```python
from build123d import *

# Parameters (mm, degrees)
SKETCH_1_R          = 27
EXTRUDE_1_DEPTH     = 45
SKETCH_2_R          = 11
CUT_EXTRUDE_1_DEPTH = 20
CUT_EXTRUDE_2_DEPTH = 20


with BuildPart() as part:
    # 草图1 → 凸台-拉伸1 (new body)
    with BuildSketch(Plane(origin=(0, 0, 0), x_dir=(1, 0, 0), z_dir=(0, 1, 0))):
        with Locations(Location((0, 0, 0), (0, 0, 90))):
            Circle(SKETCH_1_R)
    extrude(amount=EXTRUDE_1_DEPTH)

    # 草图2 → 切除-拉伸1 (cut)
    with BuildSketch(Plane(origin=(0, 45, 0), x_dir=(1, 0, 0), z_dir=(0, 1, 0))):
        with Locations(Location((0, 0, 0), (0, 0, 270))):
            Circle(SKETCH_2_R)
    extrude(amount=-CUT_EXTRUDE_1_DEPTH, mode=Mode.SUBTRACT)

    # 草图3 → 切除-拉伸2 (cut)
    with BuildSketch(Plane.XZ):
        with BuildLine():
            Line((-2.6, 10.2), (2.6, 10.2))
            Line((2.6, 10.2), (2.6, 6.499230724))
            ThreePointArc((2.6, 6.499230724), (0, -7), (-2.6, 6.499230724))
            Line((-2.6, 6.499230724), (-2.6, 10.2))
        make_face()
    extrude(amount=-CUT_EXTRUDE_2_DEPTH, mode=Mode.SUBTRACT)


solid = part.part
```
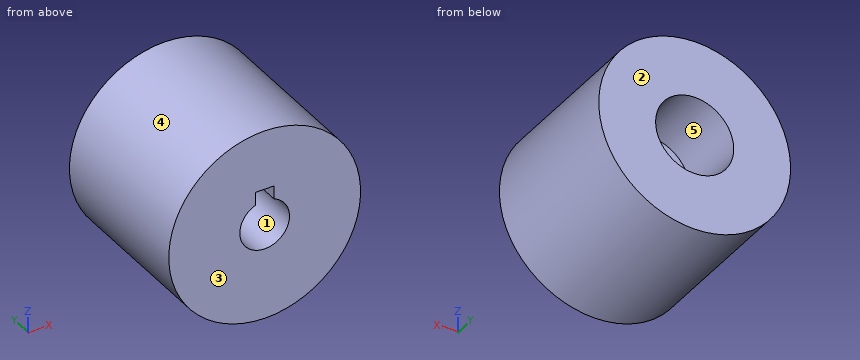
Work out the finished part from the listing and answer in its coordinate system (mm). Face numbers are marked on the shaded views. A direction names the side the tool comes from. Give positions to 0.01 mm unless a question says otherwise; leave off trailing zeros. Loops run counter-clockwise (first coordinate to the right, second up) from the corner with the lowest first, then second, coordinate; pieces in that order, holes last. Notation, with made-up numbers: (75.5, -18) - (123.5, -18) arc R26 cw to (123.5, 9) - close; hole circle Ø3 at (35, 39). An arc over 180 degrees is marked (long way). Use CSV: the item, a comma, the result in double quotes. Start each with the question number.
(1) Determine the mould class of the marked faces 3, 4 and 5 for opening direction X: released by +X, released by -X, zero draft, split by the parting line, or undercut.
(2) Find section C-C, the plane y = 14. Determine the outline of the cut face in (x, z).
(3) Find section D-D, the plane y = 36.5. Determine the outline of the cut face in (x, z).
(4) Find section A-A, the plane z = 0. Determine the outline of the cut face in (x, y), plus the area to 3 significant figures.
(5) Find the intervals of material crossed by L1, parallel to X at y = 37.5, z = 0; L2, parallel to X at y = 11.25, z = 0; L3, parallel to Y at x = -7, z = -4, in increasing order.
(6) Each of these flat-tipped pins is pushed along its axis until it touches: pin 1 (1.9 mm diameter, centred on y = 11.5, z = 8, fed in from -X); pin 2 (4 mm diameter, centred on x = -4, y = 22, fed in from -Z); pin 3 (3 mm diameter, centred on y = 6.5, z = -2.5, fed in from -X). Where does it stop, or does it pass through?
(7) A tool of negligible diameter and unlimited length cuts with its end or side. For the marked faces 1 and 2, from which of +Z, -Z, +X, -X, +Y, -Y can it reach the whole face along a straight path? Write none if from no direction.
(8) Find section B-B, the plane x = 0. Determine the outline of the cut face in (y, z), plus the area to 3 significant figures.
Results found:
1,face 3,"zero draft"
1,face 4,"split by the parting line"
1,face 5,"undercut"
2,outline,"circle Ø54 at (0, 0); hole (-2.6, 6.5) arc R7 ccw (long way) to (2.6, 6.5) - (2.6, 10.2) - (-2.6, 10.2) - close"
3,outline,"circle Ø54 at (0, 0); hole circle Ø22 at (0, 0)"
4,outline,"(-27, 0) - (-7, 0) - (-7, 20) - (7, 20) - (7, 0) - (27, 0) - (27, 45) - (11, 45) - (11, 25) - (-11, 25) - (-11, 45) - (-27, 45) - close"
4,area,"1,710 mm^2"
5,L1,"-27 to -11, 11 to 27"
5,L2,"-27 to -7, 7 to 27"
5,L3,"0 to 25"
6,pin 1,"x = -26.06"
6,pin 2,"z = -26.93"
6,pin 3,"x = -26.98"
7,face 1,"-Y"
7,face 2,"+Z, -Z, +X, -X, +Y"
8,outline,"(0, -27) - (45, -27) - (45, -11) - (25, -11) - (25, 11) - (45, 11) - (45, 27) - (0, 27) - (0, 10.2) - (20, 10.2) - (20, -7) - (0, -7) - close"
8,area,"1,650 mm^2"
